Input: part model. Units: mm. Frame: model coordinates. Face numbers are marked on the shaded views. Give positions to 0.01 mm unless a question says otherwise; leave off trailing zeros. Write each loop counter-clockwise with the first axis right and the second up, starting at its lowest first coordinate (ties: lowest second). Pieces come first, ordered by that corner, then holes. Notation, with made-up numbers: (33, -15) -> (47, -15) arc R27 ccw to (47, 6) -> close; hole circle Ø7 at (-12, 61). An arc over 180 degrees is marked (long way). Answer as a JSON object with one key per item and string values. Group by question number.
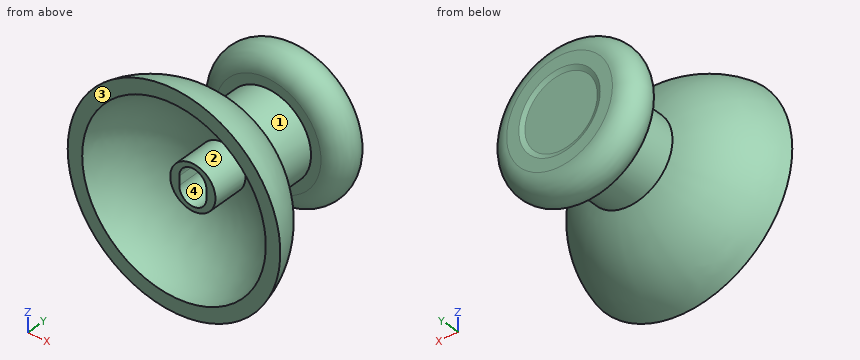
from build123d import *

# Parameters (mm, degrees)
SKETCH2_R           = 2.5
SKETCH2_R_2         = 2
SKETCH2_R_3         = 0.5
BOSS_EXTRUDE2_DEPTH = 4
CUT_EXTRUDE1_DEPTH  = 20.550319811


with BuildPart() as part:
    # Sketch1 → Revolve1 (revolve)
    with BuildSketch(Plane.XY, mode=Mode.PRIVATE) as revolve1_sk:
        with BuildLine():
            ThreePointArc((2, 6.5), (7.211992141, 4.675975116), (10.149199243, 0))
            Line((10.149199243, 0), (11.75, 0))
            ThreePointArc((11.75, 0), (9.285070189, 4.71606551), (4.75, 7.5))
            Line((4.75, 7.5), (4.75, 12.5))
            Line((4.75, 12.5), (5.85, 12.5))
            ThreePointArc((5.85, 12.5), (8, 14.65), (5.85, 16.8))
            Line((5.85, 16.8), (4.5, 16.8))
            Line((4.5, 16.8), (4, 16.6))
            Line((4, 16.6), (0, 16.6))
            Line((0, 16.6), (0, 6.5))
            Line((0, 6.5), (2, 6.5))
        make_face()
    revolve(revolve1_sk.sketch.rotate(Axis((0, 0, 0), (0, -1, 0)), 180), axis=Axis((0, 0, 0), (0, -1, 0)))

    # Sketch2 → Boss-Extrude2 (add)
    # profile 1 of 8: a face of its own
    with BuildSketch(Plane.XZ.offset(-6.5)):
        Circle(SKETCH2_R)
        Circle(SKETCH2_R_2, mode=Mode.SUBTRACT)
    # profile 2 of 8: a face of its own
    with BuildSketch(Plane.XZ.offset(-6.5)):
        with BuildLine():
            Line((-1.5, 0.5), (-1.5, -0.5))
            ThreePointArc((-1.5, -0.5), (0, -2), (1.5, -0.5))
            Line((1.5, -0.5), (1.5, 0.5))
            ThreePointArc((1.5, 0.5), (0, 2), (-1.5, 0.5))
        make_face()
        Circle(SKETCH2_R_3, mode=Mode.SUBTRACT)
    # profile 3 of 8: a face of its own
    with BuildSketch(Plane.XZ.offset(-6.5)):
        with BuildLine():
            ThreePointArc((0.5, 0), (0.353553391, 0.353553391), (0, 0.5))
            Line((0, 0.5), (0, -0.5))
            ThreePointArc((0, -0.5), (0.353553391, -0.353553391), (0.5, 0))
        make_face()
    # profile 4 of 8: a face of its own
    with BuildSketch(Plane.XZ.offset(-6.5)):
        with BuildLine():
            Line((0, -0.5), (0, 0.5))
            ThreePointArc((0, 0.5), (-0.5, 0), (0, -0.5))
        make_face()
    # profile 5 of 8: a face of its own
    with BuildSketch(Plane.XZ.offset(-6.5)):
        with BuildLine():
            ThreePointArc((-1.5, 0.5), (-1.060660172, 1.560660172), (0, 2))
            ThreePointArc((0, 2), (-2, 0), (0, -2))
            ThreePointArc((0, -2), (-1.060660172, -1.560660172), (-1.5, -0.5))
            Line((-1.5, -0.5), (-1.5, 0.5))
        make_face()
    # profile 6 of 8: a face of its own
    with BuildSketch(Plane.XZ.offset(-6.5)):
        with BuildLine():
            ThreePointArc((0.5, 0), (0.353553391, 0.353553391), (0, 0.5))
            Line((0, 0.5), (0, -0.5))
            ThreePointArc((0, -0.5), (0.353553391, -0.353553391), (0.5, 0))
        make_face()
    # profile 7 of 8: a face of its own
    with BuildSketch(Plane.XZ.offset(-6.5)):
        with BuildLine():
            Line((0, -0.5), (0, 0.5))
            ThreePointArc((0, 0.5), (-0.5, 0), (0, -0.5))
        make_face()
    # profile 8 of 8: a face of its own
    with BuildSketch(Plane.XZ.offset(-6.5)):
        with BuildLine():
            ThreePointArc((0, 2), (1.060660172, 1.560660172), (1.5, 0.5))
            Line((1.5, 0.5), (1.5, -0.5))
            ThreePointArc((1.5, -0.5), (1.060660172, -1.560660172), (0, -2))
            ThreePointArc((0, -2), (1.414213562, -1.414213562), (2, 0))
            ThreePointArc((2, 0), (1.414213562, 1.414213562), (0, 2))
        make_face()
    extrude(amount=BOSS_EXTRUDE2_DEPTH)

    # Sketch2_3 → Cut-Extrude1 (cut, through all)
    with BuildSketch(Plane.XZ.offset(-6.5)):
        with BuildLine():
            Line((1.5, 0.5), (1.5, -0.5))
            ThreePointArc((1.5, -0.5), (0, -2), (-1.5, -0.5))
            Line((-1.5, -0.5), (-1.5, 0.5))
            ThreePointArc((-1.5, 0.5), (0, 2), (1.5, 0.5))
        make_face()
    extrude(amount=CUT_EXTRUDE1_DEPTH, mode=Mode.SUBTRACT)


solid = part.part
1. Section A-A (y = 5). State how many separate pieces and enclosed holes the cut face has, plus the area to 3 significant figures.
2. Section B-B (y = 13.5). Return the cut outline in (x, z), plus the area to 3 significant figures.
3. Mould query, pull axis X, two halves, no side actions, for the marked faces 1, 2, 3 and 4. Classes: pulls with the +X half, pulls with the -X half, needs draft (parallel to the pull), parting line crosses it, or undercut.
4. Contact query for flat-ended pins moving along their axis: pin 1 Ø8 at (y, z) = (10, 3.5) entering from -X; pin 2 Ø8 at (y, z) = (2, -3.5) entering from +X; pin 3 Ø6 at (x, z) = (-3, 2.5) entering from -Y. Output: stop coordinate, or through.
5. Line query: line 1 (Z direction, x = 1.25, y = 4.25); line 2 (Y direction, x = -4.5, z = 2); line 3 (X direction, y = 4.75, z = -2.75). Output: solid intervals per line, ascending.
Working result:
{
 "1": {"separate pieces": "2", "enclosed holes": "2", "area": "120 mm^2"},
 "2": {"outline": "circle Ø15.33 at (0, 0)", "area": "185 mm^2"},
 "3": {"face 1": "parting line crosses it", "face 2": "undercut", "face 3": "needs draft", "face 4": "undercut"},
 "4": {"pin 1": "stops at x = -7.53", "pin 2": "stops at x = 11.75", "pin 3": "stops at y = 2.5"},
 "5": {"line 1": "z = -9.61 to -7.6, -2.17 to -1.33, 1.33 to 2.17, 7.6 to 9.61", "line 2": "y = 5.97 to 7.45, 12.5 to 16.8", "line 3": "x = -8.84 to -6.57, 6.57 to 8.84"}
}
